Check sheet for the drawn part. Datum: minimum x, y, z corner. Units: mm. A direction names the side the tool comes from. Round coordinates to 2 decimals unless told otherwise and drop trailing zeros. Order: outer loops, then holes, each group sorted by start corner. A loop starts at its lowest first (then second) coordinate and runs counter-clockwise, first axis right, second up. Notation, with made-up numbers: (10, 7.25) -> (51, 7.25) arc R20 cw to (51, 22.25) -> close; hole circle Ø2 at (46, -2). An arc over 180 degrees is marked (long way). Answer in a Markdown table with one row per item.
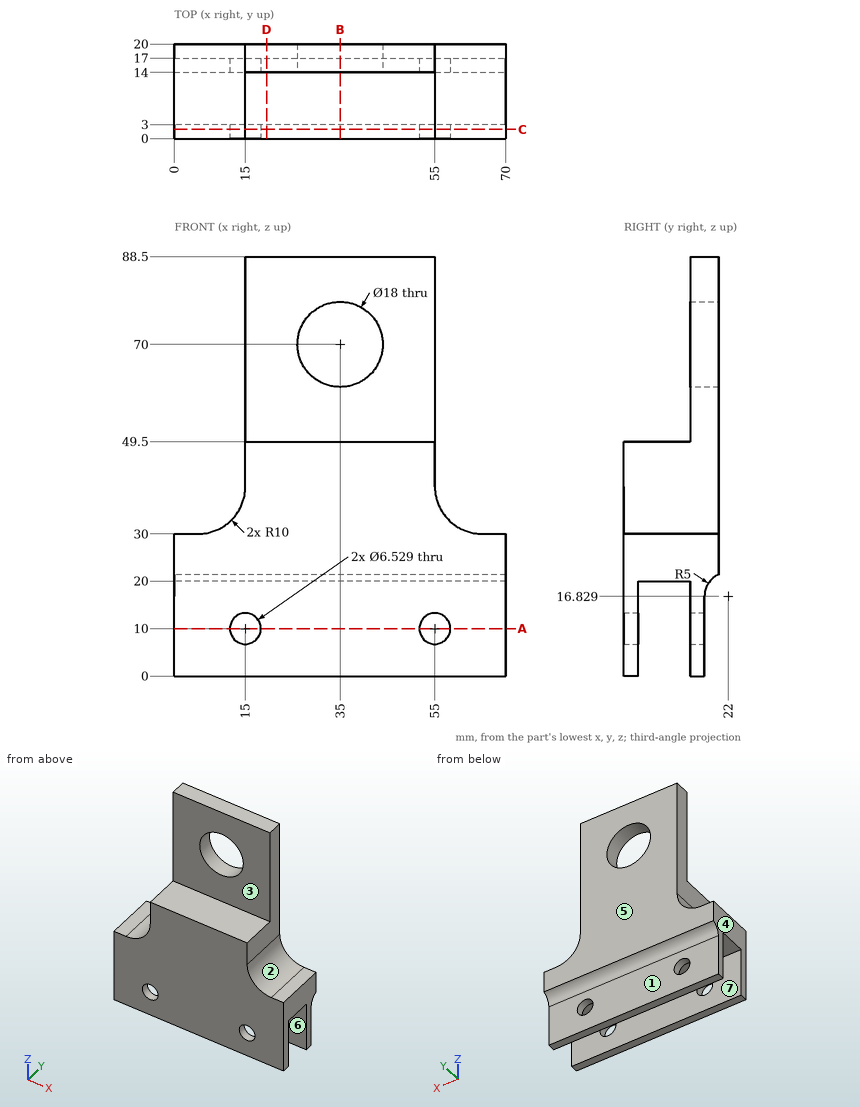
(1) Tool access check on the marked faces 1, 2 and 3. Record the directions out of +Z, -Z, +X, -X, +Y, -Y that give a thin tool (end or side, any length) a straight path to the whole face; none if there is none.
Solutions:
| item | result |
|---|---|
| face 1 | -Z, +X, -X, +Y |
| face 2 | +Z, +X, +Y, -Y |
| face 3 | +Z, +X, -X, -Y |
(2) Section check B-B on x = 35. Record the boundary of the cut face in (y, z).
Solutions:
| item | result |
|---|---|
| outline | (0, 0) -> (3, 0) -> (3, 20) -> (14, 20) -> (14, 0) -> (17, 0) -> (17, 16.83) arc R5 cw to (20, 21.41) -> (20, 61) -> (14, 61) -> (14, 49.5) -> (0, 49.5) -> close; (14, 79) -> (20, 79) -> (20, 88.5) -> (14, 88.5) -> close |
(3) Section check A-A on z = 10. Record the boundary of the cut face in (x, y) (1 decimal).
Solutions:
| item | result |
|---|---|
| outline | (0, 0) -> (11.7, 0) -> (11.7, 3) -> (0, 3) -> close; (0, 14) -> (11.7, 14) -> (11.7, 17) -> (0, 17) -> close; (18.3, 0) -> (51.7, 0) -> (51.7, 3) -> (18.3, 3) -> close; (18.3, 14) -> (51.7, 14) -> (51.7, 17) -> (18.3, 17) -> close; (58.3, 0) -> (70, 0) -> (70, 3) -> (58.3, 3) -> close; (58.3, 14) -> (70, 14) -> (70, 17) -> (58.3, 17) -> close |
(4) Depth check by flat-ended pin: pin 1 Ø4 at (x, y) = (34.5, 7.5) entering from +Z; pin 2 Ø6 at (x, z) = (24, 10) entering from +Y; pin 3 Ø10 at (y, z) = (13, 59) entering from -X. Enter the tip coordinate at first touch or a pass-through.
Solutions:
| item | result |
|---|---|
| pin 1 | z = 49.5 |
| pin 2 | y = 17 |
| pin 3 | x = 15 |
(5) Section check D-D on x = 19.5. Record the boundary of the cut face in (y, z).
Solutions:
| item | result |
|---|---|
| outline | (0, 0) -> (3, 0) -> (3, 20) -> (14, 20) -> (14, 0) -> (17, 0) -> (17, 16.83) arc R5 cw to (20, 21.41) -> (20, 88.5) -> (14, 88.5) -> (14, 49.5) -> (0, 49.5) -> close |
(6) Section check C-C on y = 2. Record the boundary of the cut face in (x, z) (1 decimal).
Solutions:
| item | result |
|---|---|
| outline | (0, 0) -> (70, 0) -> (70, 30) -> (65, 30) arc R10 cw to (55, 40) -> (55, 49.5) -> (15, 49.5) -> (15, 40) arc R10 cw to (5, 30) -> (0, 30) -> close; hole circle Ø6.5 at (15, 10); hole circle Ø6.5 at (55, 10) |
(7) Scan lines: probe 1 along X at (y, z) = (15.6, 10) (1 decimal); probe 2 along X at (y, z) = (18.2, 70); probe 3 along Y at (x, z) = (7, 8). Record each from-to range of solid material in increasing order. Write a range as from..to.
Solutions:
| item | result |
|---|---|
| probe 1 | 0..11.7, 18.3..51.7, 58.3..70 |
| probe 2 | 15..26, 44..55 |
| probe 3 | 0..3, 14..17 |
(8) Draft check along Y on the marked faces 4, 5, 6 and 7. Enter one of: pulls with the +Y half, pulls with the -Y half, needs draft (parallel to the pull), parting line crosses it, or undercut.
Solutions:
| item | result |
|---|---|
| face 4 | needs draft |
| face 5 | pulls with the +Y half |
| face 6 | undercut |
| face 7 | undercut |
